Geometry check sheet. Reference: the model listing, model coordinates, mm. A direction names the side the tool comes from. Coordinates: 2 decimals unless noted, no trailing zeros. Write each loop counter-clockwise with the first axis right and the second up, starting at its lowest first coordinate (ties: lowest second). Pieces come first, ordered by that corner, then holes. Notation, with made-up numbers: (13, 20) -> (58, 20) arc R21 cw to (58, 53) -> close; hole circle Ø11 at (5.25, 52). An arc over 180 degrees is marked (long way). Answer in a Markdown table with one row per item. Add a question column.
Q1. Tool access check on faces 4 (the face through (96.812, 1.972, 0.572)), 5 (the face through (115.724, 3.493, 0.782)), 6 (the face through (120, 1, -3)), 7 (the face through (-17, 2, 0)), 8 (the face through (75.53, 1.972, -14.353)). Record the directions out of +Z, -Z, +X, -X, +Y, -Y that give a thin tool (end or side, any length) a straight path to the whole face; none if there is none.
Q2. Gauge pin test, flat ends, axial feed: P1, Ø1.5, axis at y = 1, z = -5, coming from the -X side; P2, Ø8.5, axis at x = 121.68, z = 0, coming from the -Y side; P3, Ø6, axis at x = 120, z = 0, coming from the +Y side. Record the tip position at first contact, or that the pin passes through.
Q3. Thickness scan on line 1 (Z direction, x = 85, y = 0.25); line 2 (Z direction, x = -5, y = 2); line 3 (Z direction, x = 94, y = 2.4). Record the ranges inside material, lowest first.
Q4. Section check C-C, the plane y = 1.75. Count the separate pieces of the cut face and the enclosed holes in it, and give its area (3 significant figures).
Q5. Release check for a two-part mould opening along Z. For faces 1 (the face through (68.706, 1.972, 0.397)), 2 (the face through (133.33, 1.97, -0.25)), 3 (the face through (43, 0, -4)) record: pulls with the +Z half, pulls with the -Z half, needs draft (parallel to the pull), parting line crosses it, or undercut.
Q6. Section check A-A, the plane x = 12.5. Record the boundary of the cut face in (y, z).
Q7. Section check B-B, the plane x = 76. Record the boundary of the cut face in (y, z).
```python
from build123d import *

# Parameters (mm, degrees)
SKETCH_1_R          = 6.5
SKETCH_1_R_2        = 2.7
EXTRUDE_1_DEPTH     = 4
SKETCH_4_R          = 2
SKETCH_4_R_2        = 1.5
CUT_EXTRUDE_4_DEPTH = 135.471393041
SKETCH_5_R          = 6.01
CUT_EXTRUDE_5_DEPTH = 1
CUT_EXTRUDE_START   = -1
SKETCH_6_R          = 6.01
CUT_EXTRUDE_6_DEPTH = 1


with BuildPart() as part:
    # 草图1 → 凸台-拉伸1 (new body)
    with BuildSketch(Plane(origin=(0, 0, 0), x_dir=(1, 0, 0), z_dir=(0, 1, 0))):
        with BuildLine():
            Line((0, 16.99999971), (30, 16.99999971))
            Line((30, 16.99999971), (122.352686729, 11.63070719))
            ThreePointArc((122.352686729, 11.63070719), (133.3325, 0), (122.352686729, -11.63070719))
            Line((122.352686729, -11.63070719), (30, -16.99999971))
            Line((30, -16.99999971), (0, -16.99999971))
            ThreePointArc((0, -16.99999971), (-16.99999971, 0), (0, 16.99999971))
        make_face()
        with Locations(Location((0, 0, 0), (0, 0, 270))):
            Circle(SKETCH_1_R, mode=Mode.SUBTRACT)
        with Locations(Location((121.6825, 0, 0), (0, 0, 270))):
            Circle(SKETCH_1_R_2, mode=Mode.SUBTRACT)
        Polygon((33.501928657, 10.097744769), (52.860659349, -9.261358145), (21.859555817, -11.619111976), align=None, mode=Mode.SUBTRACT)
        Polygon((73.108054682, 7.815553359), (87.546682357, -6.623351936), (64.424639981, -8.381872691), align=None, mode=Mode.SUBTRACT)
        Polygon((79.703760078, 7.21983651), (93.560376125, -6.637045967), (100.155176587, 5.664427182), align=None, mode=Mode.SUBTRACT)
        Polygon((100.078676439, -5.670245314), (105.453109286, 4.354840622), (114.389620729, -4.581842649), align=None, mode=Mode.SUBTRACT)
        Polygon((39.307552848, 10.292124316), (67.540710691, 8.144883461), (58.436595957, -8.837286599), align=None, mode=Mode.SUBTRACT)
        Polygon((13.760637839, 10.097744769), (28.501928657, 10.097744769), (23.357153007, 0.501045083), align=None, mode=Mode.SUBTRACT)
    extrude(amount=EXTRUDE_1_DEPTH)

    # 草图4 → 切除-拉伸4 (cut, through all)
    with BuildSketch(Plane(origin=(0, 4, 0), x_dir=(1, 0, 0), z_dir=(0, 1, 0))):
        with Locations(Location((0, 10.2, 0), (0, 0, 270))):
            Circle(SKETCH_4_R)
        with Locations(Location((8.833459119, -5.1, 0), (0, 0, 270))):
            Circle(SKETCH_4_R)
        with Locations(Location((-8.833459119, -5.1, 0), (0, 0, 270))):
            Circle(SKETCH_4_R)
        with Locations(Location((-6.25, 10.825317547, 0), (0, 0, 270))):
            Circle(SKETCH_4_R_2)
        with Locations(Location((6.25, 10.825317547, 0), (0, 0, 270))):
            Circle(SKETCH_4_R_2)
        with Locations(Location((12.5, 0, 0), (0, 0, 270))):
            Circle(SKETCH_4_R_2)
        with Locations(Location((6.25, -10.825317547, 0), (0, 0, 270))):
            Circle(SKETCH_4_R_2)
        with Locations(Location((-6.25, -10.825317547, 0), (0, 0, 270))):
            Circle(SKETCH_4_R_2)
        with Locations(Location((-12.5, 0, 0), (0, 0, 270))):
            Circle(SKETCH_4_R_2)
    extrude(amount=-CUT_EXTRUDE_4_DEPTH, mode=Mode.SUBTRACT)

    # 草图5 → 切除-拉伸5 (cut)
    with BuildSketch(Plane.XZ):
        with Locations(Location((121.6825, 0, 0), (0, 0, 270))):
            Circle(SKETCH_5_R)
    extrude(amount=-CUT_EXTRUDE_5_DEPTH, mode=Mode.SUBTRACT)

    # 草图6 → 切除-拉伸6 (cut)
    with BuildSketch(Plane(origin=(0, 4, 0), x_dir=(1, 0, 0), z_dir=(0, 1, 0)).offset(CUT_EXTRUDE_START)):
        with Locations(Location((121.6825, 0, 0), (0, 0, 90))):
            Circle(SKETCH_6_R)
    extrude(amount=CUT_EXTRUDE_6_DEPTH, mode=Mode.SUBTRACT)


solid = part.part
```
Calculated:
| question | item | result |
|---|---|---|
| 1 | face 4 | +Y, -Y |
| 1 | face 5 | +Y |
| 1 | face 6 | -Y |
| 1 | face 7 | -X, +Y, -Y |
| 1 | face 8 | -Z, +X, +Y, -Y |
| 2 | P1 | stops at x = -16.46 |
| 2 | P2 | stops at y = 1 |
| 2 | P3 | stops at y = 3 |
| 3 | line 1 | z = -13.8 to -6.82, -1.92 to 4.08, 6.82 to 13.8 |
| 3 | line 2 | z = -16.25 to -11.65, -10 to -4.15, 4.15 to 10, 11.65 to 16.25 |
| 3 | line 3 | z = -13.28 to -6.13, 5.82 to 13.28 |
| 4 | separate pieces | 1 |
| 4 | enclosed holes | 17 |
| 4 | area | 3,060 mm² |
| 5 | face 1 | undercut |
| 5 | face 2 | parting line crosses it |
| 5 | face 3 | needs draft |
| 6 | outline | (0, -17) -> (4, -17) -> (4, -1.5) -> (0, -1.5) -> close; (0, 1.5) -> (4, 1.5) -> (4, 17) -> (0, 17) -> close |
| 7 | outline | (0, -14.33) -> (4, -14.33) -> (4, -4.92) -> (0, -4.92) -> close; (0, 7.5) -> (4, 7.5) -> (4, 14.33) -> (0, 14.33) -> close |
